Source: CAD feature listing. Evaluate the final solid. Frame: model axes, mm. A direction names the side the tool comes from. Coordinates: 2 decimals unless noted, no trailing zeros. Order: outer loops, then holes, each group sorted by start corner. A loop starts at its lowest first (then second) coordinate and runs counter-clockwise, first axis right, second up.
Autodesk Inventor part; units mm, degrees
ref_plane "YZ Plane" through (0, 0, 0) normal (1, 0, 0) x (0, 1, 0)
ref_plane "XZ Plane" through (0, 0, 0) normal (0, 1, 0) x (-1, 0, 0)
ref_plane "XY Plane" through (0, 0, 0) normal (0, 0, 1) x (1, 0, 0)
sketch "Sketch1" plane through (0, 0, 0) normal (0, 1, 0) x (-1, 0, 0)
  line L0 (-203.2, 0) -> (203.2, 0)
  line L1 (-200.66, 0) -> (-203.2, 0)
  line L2 (-203.2, 0) -> (-203.2, -22.86)
  line L3 (-200.66, -22.86) -> (-200.66, 0)
  line L4 (203.2, 0) -> (200.66, 0)
  line L5 (203.2, -22.86) -> (203.2, 0)
  arc A0 (-200.66, 2.54) -> (-203.2, 0) centre (-200.66, 0) ccw
  arc A1 (203.2, 0) -> (200.66, 2.54) centre (200.66, 0) ccw
  line L6 (-200.66, 2.54) -> (200.66, 2.54)
  line L7 (200.66, 0) -> (200.66, -29.21)
  line L8 (200.66, -29.21) -> (203.2, -29.21)
  line L9 (203.2, -29.21) -> (203.2, -22.86)
  line L10 (-203.2, 0) -> (-203.2, -29.21)
  line L11 (-203.2, -29.21) -> (-200.66, -29.21)
  line L12 (-200.66, -29.21) -> (-200.66, -22.86)
  line L13 (203.2, 0) -> (200.66, 0)
  point P0 (0, 0)
  dimension "d0" = 406.4
  dimension "d1" = 2.54
  dimension "d5" = 2.54
  dimension "d6" = 2.54
  dimension "d7" = 401.32
  dimension "d8" = 29.21
  dimension "d9" = 29.21
extrude "Extrusion1" add sketch "Sketch1" along normal blind 203.2
sketch "Sketch2" plane through (203.2, 0, 0) normal (1, 0, 0) x (0, 0, -1)
  circle A0 centre (13.97, 12.7) radius 6.35
  circle A1 centre (13.97, 165.1) radius 6.35
  point P0 (0, 0)
  dimension "d12" = 12.7
  dimension "d13" = 12.7
extrude "Extrusion2" cut sketch "Sketch2" against normal blind 406.4
sketch "Sketch3" plane through (-200.66, 0, 2.54) normal (0, 0, 1) x (1, 0, 0)
  line L0 (-2.54, 0) -> (-2.54, 203.2)
  line L1 (0, 203.2) -> (401.32, 203.2)
  line L2 (0, 203.2) -> (-2.54, 203.2)
  line L3 (403.86, 203.2) -> (401.32, 203.2)
  line L4 (403.86, 0) -> (403.86, 203.2)
  line L5 (0, 0) -> (401.32, 0)
  line L6 (403.86, 0) -> (401.32, 0)
  line L7 (0, 0) -> (-2.54, 0)
  line L8 (0, 177.8) -> (200.66, 177.8)
  line L9 (200.66, 177.8) -> (200.66, 203.2)
  line L10 (200.66, 203.2) -> (0, 203.2)
  line L11 (0, 177.8) -> (-2.54, 177.8)
  line L12 (-2.54, 177.8) -> (-2.54, 203.2)
  line L13 (-2.54, 203.2) -> (0, 203.2)
  line L14 (162.56, 203.2) -> (238.76, 203.2)
  line L15 (238.76, 203.2) -> (238.76, 177.8)
  line L16 (238.76, 177.8) -> (162.56, 177.8)
  line L17 (162.56, 177.8) -> (162.56, 203.2)
  point P0 (200.66, 0)
  dimension "d16" = 76.2
  dimension "d17" = 25.4
sketch "Sketch4" plane through (-200.66, 0, 2.54) normal (0, 0, 1) x (1, 0, 0)
  line L0 (0, 203.2) -> (401.32, 203.2)
  line L1 (162.558, 203.2) -> (198.118, 203.2) construction
  line L2 (264.16, 177.8002) -> (238.76, 177.8002)
  line L3 (238.76, 203.2) -> (264.1598, 177.8002)
  line L4 (264.1598, 177.8002) -> (406.3779, 177.8002)
  line L5 (403.86, 0) -> (403.86, 203.2)
  line L6 (403.86, 177.8002) -> (403.86, 203.2)
  line L7 (403.86, 203.2) -> (238.76, 203.2)
  line L8 (162.558, 177.8002) -> (137.158, 177.8002)
  line L9 (137.158, 177.8002) -> (162.558, 203.2)
  line L10 (162.558, 203.2) -> (-2.542, 203.2)
  line L11 (-2.542, 177.8002) -> (-2.542, 203.2)
  line L12 (-2.542, 203.2) -> (162.558, 203.2)
  line L13 (137.158, 177.8002) -> (-2.542, 177.8002)
  line L14 (-2.54, 0) -> (-2.54, 203.2)
  point P0 (200.66, 0)
  dimension "d21" = 25.4
  dimension "d22" = 165.1
extrude "Extrusion3" cut sketch "Sketch4" against normal blind 31.75
properties part number "4barFrontPlate"
Q1. Section query D-D on x = 20. Output: boundary loops of the cut face in (y, z), plus the area to 3 significant figures.
Solutions:
outline: (0, 0) - (203.2, 0) - (203.2, 2.54) - (0, 2.54) - close
area: 516 mm2
Q2. Set-up query: faces 4 (the cylindrical face through (201.948, 18.996, -13.143)), 5 (the flat face through (-200.66, 88, -14)), 6 (the flat face through (133, 177.8, 1)). Return all of +Z, -Z, +X, -X, +Y, -Y with unobstructed straight access to the full face (end or side cutting, diameter ignored); none if empty.
Solutions:
face 4: +X, -X
face 5: -Z, +Y, -Y
face 6: +Z, -Z, +X, +Y
Q3. Section query C-C on x = 100. Output: boundary loops of the cut face in (y, z).
Solutions:
outline: (0, 0) - (177.8, 0) - (177.8, 2.54) - (0, 2.54) - close
Q4. Pull-direction query (X, two-part tool) for faces 1 (the flat face through (3, 100, 0)), 2 (the flat face through (203.2, 88, -14)), 3 (the flat face through (-133, 177.8, 1)); classes: pulls with the +X half, pulls with the -X half, needs draft (parallel to the pull), parting line crosses it, or undercut.
Solutions:
face 1: undercut
face 2: pulls with the +X half
face 3: needs draft
Q5. Section query A-A on y = 12.7. Output: boundary loops of the cut face in (x, z), plus the area to 3 significant figures.
Solutions:
outline: (-203.2, -29.21) - (-200.66, -29.21) - (-200.66, -20.32) - (-203.2, -20.32) - close; (-203.2, -7.62) - (-200.66, -7.62) - (-200.66, 0) - (200.66, 0) - (200.66, -7.62) - (203.2, -7.62) - (203.2, 0) arc R2.54 ccw to (200.66, 2.54) - (-200.66, 2.54) arc R2.54 ccw to (-203.2, 0) - close; (200.66, -29.21) - (203.2, -29.21) - (203.2, -20.32) - (200.66, -20.32) - close
area: 1,110 mm2
Q6. Material intervals for line 1 along Y through (x, z) = (-201.2, -13.97); line 2 along X through (y, z) = (79, -19.5); line 3 along Z through (x, y) = (-201, 165), sorted ascending.
Solutions:
line 1: y = 0 to 6.35, 19.05 to 158.75, 171.45 to 177.8
line 2: x = -203.2 to -200.66, 200.66 to 203.2
line 3: z = -29.21 to -20.32, -7.62 to 2.52
Q7. Pin query (flat end, axial travel): P1, Ø10, axis at x = 136, y = 116.5, coming from the -Z side. Return the tip coordinate at first contact, or that it passes through.
Solutions:
P1: stops at z = 0
Q8. Section query B-B on z = -13.97. Output: boundary loops of the cut face in (x, y).
Solutions:
outline: (-203.2, 0) - (-200.66, 0) - (-200.66, 6.35) - (-203.2, 6.35) - close; (-203.2, 19.05) - (-200.66, 19.05) - (-200.66, 158.75) - (-203.2, 158.75) - close; (-203.2, 171.45) - (-200.66, 171.45) - (-200.66, 177.8) - (-203.2, 177.8) - close; (200.66, 0) - (203.2, 0) - (203.2, 6.35) - (200.66, 6.35) - close; (200.66, 19.05) - (203.2, 19.05) - (203.2, 158.75) - (200.66, 158.75) - close; (200.66, 171.45) - (203.2, 171.45) - (203.2, 177.8) - (200.66, 177.8) - close
